```python
from build123d import *
from build123d.topology import SkipClean

# Parameters (mm, degrees)
SKETCH1_R           = 5.35
BOSS_EXTRUDE1_DEPTH = 2.5
HOLE1_OUTLINE_R     = 1.7
HOLE1_DEPTH         = 2.5
SKETCH3_R           = 3
SKETCH3_R_2         = 1.7
BOSS_EXTRUDE2_DEPTH = 10
FILLET1_R           = 0.1
BOSS_EXTRUDE3_DEPTH = 1.5
SKETCH8_R           = 0.75
CUT_EXTRUDE1_DEPTH  = 13.539736839
CUT_EXTRUDE3_START  = -0.5
SKETCH13_R          = 1.25
CUT_EXTRUDE3_DEPTH  = 7
CHAMFER1_SIZE       = 0.25
CUT_EXTRUDE4_START  = -0.5
CUT_EXTRUDE4_DEPTH  = 0.5
FILLET2_R           = 0.4
CUT_EXTRUDE5_START  = -4.5
SKETCH15_R          = 3
CUT_EXTRUDE5_DEPTH  = 4.5


# Read off the part's stored shape, not the designer's step: Hole1
with BuildPart() as part:
    # Sketch1 → Boss-Extrude1 (new body)
    with BuildSketch(Plane(origin=(0, 0, 0), x_dir=(1, 0, 0), z_dir=(0, 1, 0))):
        with Locations(Location((0, 0, 0), (0, 0, 270))):
            Circle(SKETCH1_R)
    extrude(amount=BOSS_EXTRUDE1_DEPTH)

    # Hole1 outline → Hole1 (cut)
    with BuildSketch(Plane(origin=(0, 0, 0), x_dir=(1, 0, 0), z_dir=(0, 1, 0))):
        Circle(HOLE1_OUTLINE_R)
    extrude(amount=HOLE1_DEPTH, mode=Mode.SUBTRACT)

    # Sketch3 → Boss-Extrude2 (add)
    with BuildSketch(Plane(origin=(0, 2.5, 0), x_dir=(1, 0, 0), z_dir=(0, 1, 0))):
        with Locations(Location((0, 0, 0), (0, 0, 270))):
            Circle(SKETCH3_R)
        with Locations(Location((0, 0, 0), (0, 0, 270))):
            Circle(SKETCH3_R_2, mode=Mode.SUBTRACT)
    extrude(amount=BOSS_EXTRUDE2_DEPTH)

    # Fillet1
    fillet1_edges = [part.edges().sort_by_distance(p)[0] for p in [
        (0, 12.5, -3),
    ]]
    fillet(fillet1_edges, radius=FILLET1_R)

    # Sketch5 → Boss-Extrude3 (add)
    with BuildSketch(Plane(origin=(0, 2.5, 0), x_dir=(1, 0, 0), z_dir=(0, 1, 0))):
        with BuildLine():
            Line((-0.75, 5.297169055), (-0.75, 2.90473751))
            ThreePointArc((-0.75, 2.90473751), (0, 3), (0.75, 2.90473751))
            Line((0.75, 2.90473751), (0.75, 5.297169055))
            ThreePointArc((0.75, 5.297169055), (0, 5.35), (-0.75, 5.297169055))
        make_face()
    boss_extrude3 = extrude(amount=BOSS_EXTRUDE3_DEPTH)

    # Mirror1: Boss-Extrude3 across plane
    with SkipClean():  # the faces are left unmerged after this step: merging them gives an invalid solid
        add(boss_extrude3.mirror(Plane.XY))

    # Sketch8 → Cut-Extrude1 (cut, through all)
    with SkipClean():  # the faces are left unmerged after this step: merging them gives an invalid solid
        with BuildSketch(Plane(origin=(0, 2.5, 0), x_dir=(1, 0, 0), z_dir=(0, 1, 0))):
            with Locations(Location((3.8, 0, 0), (0, 0, 270))):
                Circle(SKETCH8_R)
            with Locations(Location((-1.9, -3.290896534, 0), (0, 0, 270))):
                Circle(SKETCH8_R)
            with Locations(Location((-1.9, 3.290896534, 0), (0, 0, 270))):
                Circle(SKETCH8_R)
        extrude(amount=-CUT_EXTRUDE1_DEPTH, mode=Mode.SUBTRACT)

    # Sketch13 → Cut-Extrude3 (cut)
    with SkipClean():  # the faces are left unmerged after this step: merging them gives an invalid solid
        with BuildSketch(Plane(origin=(0, 2.5, 0), x_dir=(1, 0, 0), z_dir=(0, 1, 0)).offset(CUT_EXTRUDE3_START)):
            with Locations(Location((-1.9, 3.290896534, 0), (0, 0, 23.073918066))):
                Circle(SKETCH13_R)
            with Locations(Location((-1.9, -3.290896534, 0), (0, 0, 102.514591278))):
                Circle(SKETCH13_R)
            with Locations(Location((3.8, 0, 0), (0, 0, 137.485408722))):
                Circle(SKETCH13_R)
        extrude(amount=CUT_EXTRUDE3_DEPTH, mode=Mode.SUBTRACT)

    # Chamfer1
    chamfer1_edges = [part.edges().sort_by_distance(p)[0] for p in [
        (-1.275, 9, -2.20836478),
        (-1.275, 9, 2.20836478),
        (2.55, 9, 0),
    ]]
    chamfer(chamfer1_edges, length=CHAMFER1_SIZE)

    # Sketch14 → Cut-Extrude4 (cut)
    with BuildSketch(Plane(origin=(0, 2.5, 0), x_dir=(1, 0, 0), z_dir=(0, 1, 0)).offset(CUT_EXTRUDE4_START)):
        with BuildLine():
            Line((-0.75, -3.780794483), (-0.75, -5.297169055))
            ThreePointArc((-0.75, -5.297169055), (-2.563606422, -4.695787699), (-4.050222345, -3.495454041))
            Line((-4.050222345, -3.495454041), (-2.716694869, -2.344582902))
            ThreePointArc((-2.716694869, -2.344582902), (-2.637189937, -4.300377092), (-0.75, -3.780794483))
        make_face()
        with BuildLine():
            Line((-0.75, 5.297169055), (-0.75, 3.780794483))
            ThreePointArc((-0.75, 3.780794483), (-2.637189937, 4.300377092), (-2.716694869, 2.344582902))
            Line((-2.716694869, 2.344582902), (-4.050222345, 3.495454041))
            ThreePointArc((-4.050222345, 3.495454041), (-2.563606422, 4.695787699), (-0.75, 5.297169055))
        make_face()
        with BuildLine():
            Line((3.388815789, -1.18043532), (5.05226317, -1.759868421))
            ThreePointArc((5.05226317, -1.759868421), (5.35, 0), (5.05226317, 1.759868421))
            Line((5.05226317, 1.759868421), (3.388815789, 1.18043532))
            ThreePointArc((3.388815789, 1.18043532), (5.05, 0), (3.388815789, -1.18043532))
        make_face()
    extrude(amount=CUT_EXTRUDE4_DEPTH, mode=Mode.SUBTRACT)

    # Fillet2
    fillet2_edges = [part.edges().sort_by_distance(p)[0] for p in [
        (-4.050222345, 2.25, -3.495454041),
        (-4.050222345, 2.25, 3.495454041),
        (5.05226317, 2.25, -1.759868421),
        (5.05226317, 2.25, 1.759868421),
    ]]
    fillet(fillet2_edges, radius=FILLET2_R)

    # Sketch15 → Cut-Extrude5 (cut)
    with BuildSketch(Plane(origin=(0, 12.5, 0), x_dir=(1, 0, 0), z_dir=(0, 1, 0)).offset(CUT_EXTRUDE5_START)):
        Circle(SKETCH15_R)
    extrude(amount=CUT_EXTRUDE5_DEPTH, mode=Mode.SUBTRACT)


solid = part.part
```
Geometry: final body of the model. Coordinates: model frame, mm. A direction names the side the tool comes from. Coordinates: 2 decimals unless noted, no trailing zeros. Order: outer loops, then holes, each group sorted by start corner. A loop starts at its lowest first (then second) coordinate and runs counter-clockwise, first axis right, second up. Notation, with made-up numbers: (10.25, 79) -> (21.25, 79) arc R18 cw to (21.25, 102) -> close; hole circle Ø10 at (2, 57.5). An arc over 180 degrees is marked (long way). Answer in a Markdown table with one row per item.
Item 1: Contact query for flat-ended pins moving along their axis: P1, Ø1.4, axis at x = -1.9, z = 3.29, coming from the -Y side; P2, Ø1.3, axis at x = 2.5, z = -4, coming from the +Y side; P3, Ø1.7, axis at x = 3.8, z = 0, coming from the +Y side; P4, Ø1.7, axis at x = 0, z = -4.5, coming from the +Y side. Output: stop coordinate, or through.
Return value:
| item | result |
|---|---|
| P1 | passes through |
| P2 | stops at y = 2.5 |
| P3 | stops at y = 2 |
| P4 | stops at y = 4 |
Item 2: Ray query, L1, parallel to Z at x = 0, y = 3.75; L2, parallel to X at y = 5, z = 0; L3, parallel to Y at x = 1, z = 3. Return the intervals inside material, ascending.
Return value:
| item | result |
|---|---|
| L1 | z = -5.35 to -1.7, 1.7 to 5.35 |
| L2 | x = -3 to -1.7, 1.7 to 2.55 |
| L3 | y = 0 to 2.5 |
Item 3: Draft query along Z for faces 4 (the cylindrical face through (0.63, 3.94, 1.58)), 5 (the flat face through (3, 2.5, -3)), 6 (the cylindrical face through (-3, 5, 0)). Return one class per face: released by +Z, released by -Z, zero draft, split by the parting line, or undercut.
Return value:
| item | result |
|---|---|
| face 4 | undercut |
| face 5 | zero draft |
| face 6 | split by the parting line |
Item 4: Section B-B on z = 0. Output: boundary loops of the cut face in (x, y).
Return value:
| item | result |
|---|---|
| outline | (-5.35, 0) -> (-1.7, 0) -> (-1.7, 8) -> (-3, 8) -> (-3, 2.5) -> (-5.35, 2.5) -> close; (1.7, 0) -> (3.05, 0) -> (3.05, 2) -> (2.55, 2) -> (2.55, 8) -> (1.7, 8) -> close; (4.55, 0) -> (5.35, 0) -> (5.35, 2) -> (4.55, 2) -> close |
Item 5: Access query for faces 1 (the cylindrical face through (2.55, 4.96, -0.02)), 2 (the cylindrical face through (-1.18, 4.96, -2.27)), 3 (the flat face through (0.75, 3, 4)). Directions: +Z, -Z, +X, -X, +Y, -Y. A direction counts if a zero-diameter tool reaches every point of the face in a straight line with its end or side. Return the directions, or none.
Return value:
| item | result |
|---|---|
| face 1 | +X, +Y |
| face 2 | +Y |
| face 3 | +Z, +X, +Y |
Item 6: Section A-A on y = 3. Output: boundary loops of the cut face in (x, z).
Return value:
| item | result |
|---|---|
| outline | (-2.17, -2.07) arc R1.25 cw to (-0.75, -3.78) -> (-0.75, -5.3) arc R5.35 ccw to (0.75, -5.3) -> (0.75, -2.9) arc R3 ccw to (2.88, -0.84) arc R1.25 cw to (2.88, 0.84) arc R3 ccw to (0.75, 2.9) -> (0.75, 5.3) arc R5.35 ccw to (-0.75, 5.3) -> (-0.75, 3.78) arc R1.25 cw to (-2.17, 2.07) arc R3 ccw to start; hole circle Ø3.4 at (0, 0) |
Item 7: Section D-D on x = -1.9. Output: boundary loops of the cut face in (y, z).
Return value:
| item | result |
|---|---|
| outline | (0, -5) -> (2, -5) -> (2, -4.04) -> (0, -4.04) -> close; (0, -2.54) -> (2, -2.54) -> (2, -2.04) -> (8, -2.04) -> (8, 2.04) -> (2, 2.04) -> (2, 2.54) -> (0, 2.54) -> close; (0, 4.04) -> (2, 4.04) -> (2, 5) -> (0, 5) -> close |
Item 8: Section C-C on x = 3.8. Output: boundary loops of the cut face in (y, z).
Return value:
| item | result |
|---|---|
| outline | (0, -3.77) -> (2.5, -3.77) -> (2.5, -1.32) -> (2, -1.32) -> (2, -0.75) -> (0, -0.75) -> close; (0, 0.75) -> (2, 0.75) -> (2, 1.32) -> (2.5, 1.32) -> (2.5, 3.77) -> (0, 3.77) -> close |
